```python
from build123d import *

# Parameters (mm, degrees)
EXTRUDE_1_DEPTH        = 4
EXTRUDE_1010_DEPTH     = 2
FILLET_1_R             = 0.25
FILLET_1_OF_MIRROR_1_R = 0.25
SKETCH_4_R             = 6
CUT_EXTRUDE_2_DEPTH    = 53.927628586


with BuildPart() as part:
    # Sketch 1 → Extrude 1 (new body)
    with BuildSketch(Plane(origin=(0, 0, 0), x_dir=(1, 0, 0), z_dir=(0, 1, 0))):
        with BuildLine():
            ThreePointArc((38.61, 30), (38.317106781, 30.707106781), (37.61, 31))
            Line((37.61, 31), (-38.61, 31))
            ThreePointArc((-38.61, 31), (-29.704013367, 16.623426496), (-26.595290936, 0))
            Line((-26.595290936, 0), (38.61, 0))
            Line((38.61, 0), (38.61, 30))
        make_face()
        with BuildLine():
            Line((38.61, 0), (-26.595290936, 0))
            ThreePointArc((-26.595290936, 0), (-29.704013367, -16.623426496), (-38.61, -31))
            Line((-38.61, -31), (37.61, -31))
            ThreePointArc((37.61, -31), (38.317106781, -30.707106781), (38.61, -30))
            Line((38.61, -30), (38.61, 0))
        make_face()
    extrude(amount=EXTRUDE_1_DEPTH)

    # Sketch 3 → Extrude 1010 (add, symmetric)
    with BuildSketch(Plane(origin=(-21.39, 0, 0), x_dir=(0, 0, -1), z_dir=(1, 0, 0))):
        Polygon((-31, 4), (-31, 12), (-33, 12), (-29, 16), (-29, 4), align=None)
    extrude_1010 = extrude(amount=EXTRUDE_1010_DEPTH, both=True)

    # Fillet 1
    fillet_1_edges = [part.edges().sort_by_distance(p)[0] for p in [
        (-21.39, 12, 33),
        (-21.39, 16, 29),
    ]]
    fillet(fillet_1_edges, radius=FILLET_1_R)

    # Mirror 1: Extrude 1010 across plane
    add(extrude_1010.mirror(Plane.XY))

    # Fillet 1 of Mirror 1
    fillet_1_of_mirror_1_edges = [part.edges().sort_by_distance(p)[0] for p in [
        (-21.39, 12, -33),
        (-21.39, 16, -29),
    ]]
    fillet(fillet_1_of_mirror_1_edges, radius=FILLET_1_OF_MIRROR_1_R)

    # Sketch 4 → Cut-Extrude 2 (cut, through all)
    with BuildSketch(Plane.XZ):
        with Locations(Location((28.61, 0, 0), (0, 0, 270))):
            Circle(SKETCH_4_R)
    extrude(amount=-CUT_EXTRUDE_2_DEPTH, mode=Mode.SUBTRACT)


solid = part.part
```
Input: part model. Units: mm. Frame: model coordinates. A direction names the side the tool comes from. Give positions to 0.01 mm unless a question says otherwise; leave off trailing zeros. Loops run counter-clockwise (first coordinate to the right, second up) from the corner with the lowest first, then second, coordinate; pieces in that order, holes last.
1) Section query C-C on x = -12.5. Return the cut outline in (y, z), and give its area (3 significant figures).
A:
outline: (0, -31) - (4, -31) - (4, 31) - (0, 31) - close
area: 248 mm2
2) Line query: L1, parallel to X at y = 1.75, z = 0; L2, parallel to Z at x = -21, y = 6.5; L3, parallel to Y at x = 22.5, z = -14.5. Output: solid intervals per line, ascending.
A:
L1: x = -26.6 to 22.61, 34.61 to 38.61
L2: z = -31 to -29, 29 to 31
L3: y = 0 to 4
3) Section query A-A on x = 28.61. Return the cut outline in (y, z), and give its area (3 significant figures).
A:
outline: (0, -31) - (4, -31) - (4, -6) - (0, -6) - close; (0, 6) - (4, 6) - (4, 31) - (0, 31) - close
area: 200 mm2
4) Reachability of faces 1 (the flat face through (-4, 3, 31)), 2 (the flat face through (-21, 10, 29)), 3 (the flat face through (-23.39, 10, 30)), 4 (the flat face through (-21, 14, 31)), 5 (the flat face through (-19.39, 10, 30)) from +Z, -Z, +X, -X, +Y, -Y: full face, straight path, thin tool, end or side. Return the list, or none.
A:
face 1: +Z, +X, -X, -Y
face 2: +X, -X, +Y
face 3: +Z, -Z, -X, +Y
face 4: +Z, +X, -X, +Y
face 5: +Z, -Z, +X, +Y
5) Mould query, pull axis X, two halves, no side actions, for faces 6 (the flat face through (-23.39, 10, -30)), 7 (the cylindrical face through (34.56, 1.97, 0.78)), 8 (the flat face through (-3, 3, -31)). Classes: released by +X, released by -X, zero draft, split by the parting line, or undercut.
A:
face 6: released by -X
face 7: undercut
face 8: zero draft
6) Section query B-B on y = 6.5. Return the cut outline in (x, z).
A:
outline: (-23.39, -31) - (-19.39, -31) - (-19.39, -29) - (-23.39, -29) - close; (-23.39, 29) - (-19.39, 29) - (-19.39, 31) - (-23.39, 31) - close
7) Section query D-D on z = -18.5. Return the cut outline in (x, y), and give its area (3 significant figures).
A:
outline: (-30.48, 0) - (38.61, 0) - (38.61, 4) - (-30.48, 4) - close
area: 276 mm2
8) Contact query for flat-ended pins moving along their axis: pin 1 (4 mm diameter, centred on y = 11, z = -30.5, fed in from -X); pin 2 (4 mm diameter, centred on y = 11.5, z = -31.5, fed in from +X); pin 3 (4.5 mm diameter, centred on x = -22.5, y = 8.5, fed in from -Z). Output: stop coordinate, or through.
A:
pin 1: stops at x = -23.39
pin 2: stops at x = -19.39
pin 3: stops at z = -31
